Job drawing, mm, ordinate dimensions from the low corner. One solid piece. A direction names the side the tool comes from. Round coordinates to 2 decimals unless told otherwise and drop trailing zeros. Loops run counter-clockwise (first coordinate to the right, second up) from the corner with the lowest first, then second, coordinate; pieces in that order, holes last.
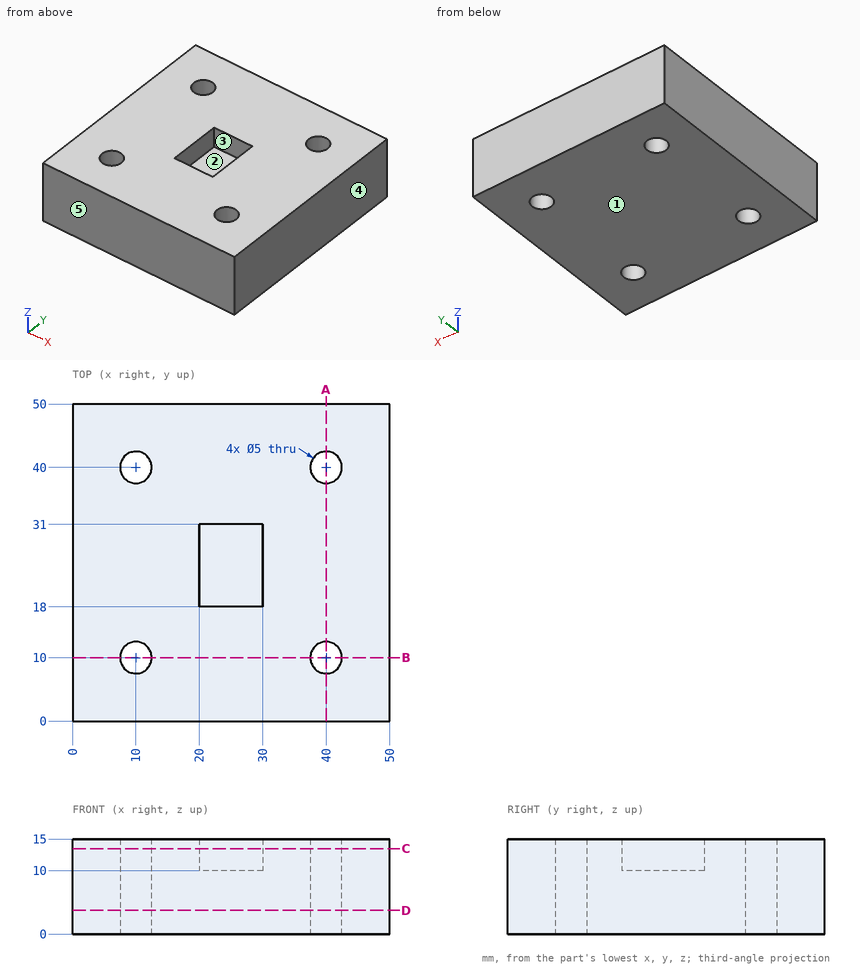
1) Wall check: line 1 along Y through (x, z) = (10, 8.5); line 2 along Y through (x, z) = (42, 8.5); line 3 along X through (y, z) = (9, 11.25). Give the ranges that are in metal, low to high.
Values:
line 1: y = 0 to 7.5, 12.5 to 37.5, 42.5 to 50
line 2: y = 0 to 8.5, 11.5 to 38.5, 41.5 to 50
line 3: x = 0 to 7.71, 12.29 to 37.71, 42.29 to 50
2) Slice it at C-C, the plane z = 13.5. Give the cut face in (x, y).
Values:
outline: (0, 0) - (50, 0) - (50, 50) - (0, 50) - close; hole circle Ø5 at (10, 10); hole circle Ø5 at (10, 40); hole (20, 18) - (30, 18) - (30, 31) - (20, 31) - close; hole circle Ø5 at (40, 10); hole circle Ø5 at (40, 40)
3) Drop a flat-ended pin along its axis: pin 1 Ø1.5 at (x, y) = (26, 23) entering from +Z. Give the stop position or say it passes through.
Values:
pin 1: stops at z = 10
4) Slice it at D-D, the plane z = 3.75. Give the cut face in (x, y), then the cut area to 3 significant figures.
Values:
outline: (0, 0) - (50, 0) - (50, 50) - (0, 50) - close; hole circle Ø5 at (10, 10); hole circle Ø5 at (10, 40); hole circle Ø5 at (40, 10); hole circle Ø5 at (40, 40)
area: 2,420 mm2
5) Slice it at A-A, the plane x = 40. Give the cut face in (y, z), then the cut area to 3 significant figures.
Values:
outline: (0, 0) - (7.5, 0) - (7.5, 15) - (0, 15) - close; (12.5, 0) - (37.5, 0) - (37.5, 15) - (12.5, 15) - close; (42.5, 0) - (50, 0) - (50, 15) - (42.5, 15) - close
area: 600 mm2
6) Tool access for the marked faces 1 and 2: list every direction of +Z, -Z, +X, -X, +Y, -Y with a clear straight run to the whole face (end or side of a thin tool).
Values:
face 1: -Z, +X, -X, +Y, -Y
face 2: +Z
7) Mould opens along Y. For the marked faces 3, 4 and 5 say: released by +Y, released by -Y, zero draft, split by the parting line, or undercut.
Values:
face 3: undercut
face 4: zero draft
face 5: released by -Y
